Input: part model. Units: mm. Frame: model coordinates. Face numbers are marked on the shaded views. A direction names the side the tool comes from. Give positions to 0.01 mm unless a question says otherwise; leave off trailing zeros. Write each loop counter-clockwise with the first axis right and the second up, starting at its lowest first coordinate (ties: lowest second). Pieces come first, ordered by that corner, then holes. Notation, with made-up numbers: (24, -29.5) - (69, -29.5) arc R13 cw to (69, -21.5) - close; hole circle Ø5 at (17.25, 69.25). An arc over 180 degrees is marked (long way). Use a Markdown table: item, result. Add a question column.
1. Section query D-D, the plane z = 2.85. Return loops of the section in (x, y), plus the area to 3 significant figures.
2. Mould query, pull axis X, two halves, no side actions, for the marked faces 3, 4 and 5. Classes: released by +X, released by -X, zero draft, split by the parting line, or undercut.
3. Set-up query: the marked faces 1 and 2. Return all of +Z, -Z, +X, -X, +Y, -Y with unobstructed straight access to the full face (end or side cutting, diameter ignored); none if empty.
4. Section query A-A, the plane x = 0. Return loops of the section in (y, z), plus the area to 3 significant figures.
5. Pin query (flat end, axial travel): pin 1 (1 mm diameter, centred on x = -14.5, z = 3.5, fed in from -Y); pin 2 (12.5 mm diameter, centred on x = 8, y = -5, fed in from +Z); pin 3 (2.5 mm diameter, centred on x = 0, y = 0, fed in from -Z); pin 4 (1.1 mm diameter, centred on x = -14.5, z = 0.5, fed in from +Y). Return the tip coordinate at first contact, or that it passes through.
6. Section query C-C, the plane y = 6.5. Return loops of the section in (x, z), plus the area to 3 significant figures.
7. Material intervals for probe 1 along Y at (x, z) = (17, 0.6); probe 2 along X at (y, z) = (1, 0.55); probe 3 along Y at (x, z) = (0, 2), sorted ascending.
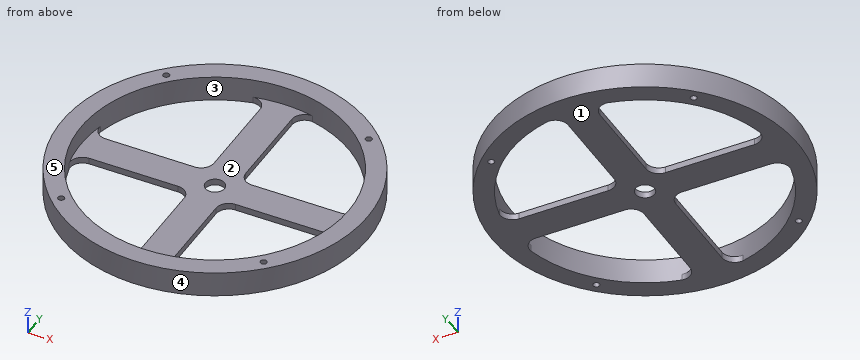
Autodesk Fusion 360 part; units mm, degrees
sketch "Sketch1" plane through (0, 0, 0) normal (0, 0, 1) x (1, 0, 0)
  circle A0 centre (0, 0) radius 24
  circle A1 centre (0, 0) radius 21
  line L0 (-2.5, 4.5) -> (-2.5, 18.4793)
  line L1 (2.5, 18.4793) -> (2.5, 4.5)
  line L2 (4.5, 2.5) -> (18.4795, 2.5)
  line L3 (18.4604, -2.5) -> (4.5, -2.5)
  line L4 (-2.5, -4.5) -> (-2.5, -18.4675)
  line L5 (2.5, -18.4675) -> (2.5, -4.5)
  line L6 (-4.5, 2.5) -> (-18.4663, 2.5)
  line L7 (-18.4663, -2.5) -> (-4.5, -2.5)
  arc A2 (2.5, 4.5) -> (4.5, 2.5) centre (4.5, 4.5) ccw
  arc A3 (4.5, -2.5) -> (2.5, -4.5) centre (4.5, -4.5) ccw
  arc A4 (-2.5, -4.5) -> (-4.5, -2.5) centre (-4.5, -4.5) ccw
  arc A5 (-4.5, 2.5) -> (-2.5, 4.5) centre (-4.5, 4.5) ccw
  line L8 (4.8374, 20.4506) -> (4.5763, 20.4953)
  line L9 (-4.8374, 20.4506) -> (-4.5763, 20.4953)
  arc A6 (-2.5, 18.4793) -> (-4.8374, 20.4506) centre (-4.5, 18.4793) ccw
  arc A7 (4.8374, 20.4506) -> (2.5, 18.4793) centre (4.5, 18.4793) ccw
  line L10 (20.4509, 4.8372) -> (20.4962, 4.5723)
  line L11 (20.4291, -4.8528) -> (20.4213, -4.8958)
  arc A8 (20.4291, -4.8528) -> (18.4604, -2.5) centre (18.4604, -4.5) ccw
  arc A9 (18.4795, 2.5) -> (20.4509, 4.8372) centre (18.4795, 4.5) ccw
  line L12 (4.847, -20.4372) -> (4.7758, -20.4497)
  line L13 (-4.847, -20.4372) -> (-4.7758, -20.4497)
  arc A10 (-4.847, -20.4372) -> (-2.5, -18.4675) centre (-4.5, -18.4675) ccw
  arc A11 (2.5, -18.4675) -> (4.847, -20.4372) centre (4.5, -18.4675) ccw
  line L14 (-20.4358, 4.848) -> (-20.4448, 4.797)
  line L15 (-20.4358, -4.848) -> (-20.4448, -4.797)
  arc A12 (-18.4663, -2.5) -> (-20.4358, -4.848) centre (-18.4663, -4.5) ccw
  arc A13 (-20.4358, 4.848) -> (-18.4663, 2.5) centre (-18.4663, 4.5) ccw
  circle A14 centre (0, 0) radius 1.5
  dimension "d1" = 48
  dimension "d2" = 42
  dimension "d6" = 2
  dimension "d7" = 2
  dimension "d8" = 2
  dimension "d9" = 2
  dimension "d10" = 2
  dimension "d11" = 2
  dimension "d12" = 2
  dimension "d13" = 2
  dimension "d14" = 2
  dimension "d15" = 2
  dimension "d16" = 2
  dimension "d17" = 2
  dimension "d18" = 3
extrude "Extrude1" add sketch "Sketch1" along normal blind 1 contours A1 L0 L1 L2 L3 L4 L5 L6 L7 A2 A3 A4 A5 A6 A7 L11 A8 A9 A10 A11 A12 A13
sketch "Sketch2" plane through (0, 0, 0) normal (0, 0, 1) x (1, 0, 0)
  circle A0 centre (0, 0) radius 21
  circle A1 centre (0, 0) radius 24
  line L0 (0, 0) -> (21, 0) construction
  line L1 (0, 0) -> (22.5, 0) construction
  circle A2 centre (15.9099, 15.9099) radius 0.5
  circle A3 centre (15.9099, -15.9099) radius 0.5
  circle A4 centre (-15.9099, -15.9099) radius 0.5
  circle A5 centre (-15.9099, 15.9099) radius 0.5
  dimension "d21" = 42
  dimension "d22" = 48
  dimension "d26" = 1
  dimension "d27" = 1
  dimension "d28" = 1
  dimension "d29" = 1
extrude "Extrude2" add sketch "Sketch2" along normal blind 4
Result sheet:
| question | item | result |
|---|---|---|
| 1 | outline | circle Ø48 at (0, 0); hole circle Ø42 at (0, 0); hole circle Ø1 at (-15.91, -15.91); hole circle Ø1 at (-15.91, 15.91); hole circle Ø1 at (15.91, -15.91); hole circle Ø1 at (15.91, 15.91) |
| 1 | area | 421 mm² |
| 2 | face 3 | undercut |
| 2 | face 4 | split by the parting line |
| 2 | face 5 | zero draft |
| 3 | face 1 | -Z, +X, -X, +Y, -Y |
| 3 | face 2 | +Z |
| 4 | outline | (-24, 0) - (-1.5, 0) - (-1.5, 1) - (-21, 1) - (-21, 4) - (-24, 4) - close; (1.5, 0) - (24, 0) - (24, 4) - (21, 4) - (21, 1) - (1.5, 1) - close |
| 4 | area | 63.0 mm² |
| 5 | pin 1 | stops at y = -19.49 |
| 5 | pin 2 | stops at z = 1 |
| 5 | pin 3 | passes through |
| 5 | pin 4 | stops at y = 19.53 |
| 6 | outline | (-23.1, 0) - (-19.97, 0) - (-19.97, 4) - (-23.1, 4) - close; (-2.5, 0) - (2.5, 0) - (2.5, 1) - (-2.5, 1) - close; (19.97, 0) - (23.1, 0) - (23.1, 4) - (19.97, 4) - close |
| 6 | area | 30.1 mm² |
| 7 | probe 1 | y = -16.94 to -12.33, -2.5 to 2.5, 12.33 to 16.94 |
| 7 | probe 2 | x = -23.98 to -1.12, 1.12 to 23.98 |
| 7 | probe 3 | y = -24 to -21, 21 to 24 |
